Here's how the part is built. I have some questions about the finished solid (model axes, mm). A direction names the side the tool comes from. Coordinates: 2 decimals unless noted, no trailing zeros. Write each loop counter-clockwise with the first axis right and the second up, starting at its lowest first coordinate (ties: lowest second). Pieces come first, ordered by that corner, then holes.
Item 1: For faces 5 (the face through (8.25, 5.24, -0.07)), 6 (the face through (11, 16, -5)), 7 (the face through (-5, 16, 10)), which set-ups out of +Z, -Z, +X, -X, +Y, -Y let a thin tool reach every point of the face, with its end or its side?
Item 2: We'd pull the mould along X, two halves only. Please class faces 1 (the face through (-11, 16, 5)), 2 (the face through (-9.59, 22.48, -0.07)), 3 (the face through (11.49, 13.1, -0.07)), 4 (the face through (-11.46, 12.87, -0.07)): +X half, -X half, draft (parallel to the pull), parting line (faces both ways), or undercut.
Item 3: If we section it at A-A (y = -2.5): Please give me the cut outline in (x, z).
Item 4: If we section it at D-D (z = 6.25): Please give me the cut outline in (x, y).
Item 5: If we section it at B-B (x = 0): Please give me the cut outline in (y, z), then the cut area to 3 significant figures.
Item 6: If we section it at C-C (y = 13): Please give me the cut outline in (x, z).
Item 7: I'm going to push flat-ended pins straight in: pin 1 Ø2 at (y, z) = (15.5, 2) entering from +X; pin 2 Ø1.2 at (y, z) = (11, 10.5) entering from +X; pin 3 Ø0.8 at (y, z) = (18, 10) entering from -X. Where does each tip first touch, or does it pass through?
Item 8: If I drill on line 1 (Z direction, x = 0, y = 2.3); line 2 (Y direction, x = 5.5, z = 7); line 3 (X direction, y = 21, z = 4.5), over which ranges is the centre line in solid material (lowest first)?
from build123d import *

# Parameters (mm, degrees)
EXTRUDE_1582_DEPTH      = 11
EXTRUDE_1582_DEPTH_BACK = 11
EXTRUDE_2052_DEPTH      = 5
EXTRUDE_2052_DEPTH_BACK = 5
EXTRUDE_2225_DEPTH      = 5
EXTRUDE_2225_DEPTH_BACK = 5
CUT_EXTRUDE_2419_REACH  = 32.666
SKETCH_4_R              = 3.5
EXTRUDE_5_DEPTH         = 22


with BuildPart() as part:
    # Эскиз1 → Extrude 1582 (new, two sides: drawn at the far end of the back side and taken through both)
    with BuildSketch(Plane.XY.offset(-EXTRUDE_1582_DEPTH_BACK)):
        with BuildLine():
            Line((9, 0), (-9, 0))
            ThreePointArc((-9, 0), (-9.662499048, 0.250937245), (-9.992506725, 0.877809978))
            Line((-9.992506725, 0.877809978), (-10.5, 5))
            Line((-10.5, 5), (10.5, 5))
            Line((10.5, 5), (9.992506725, 0.877809978))
            ThreePointArc((9.992506725, 0.877809978), (9.662499048, 0.250937245), (9, 0))
        make_face()
    extrude(amount=EXTRUDE_1582_DEPTH + EXTRUDE_1582_DEPTH_BACK)

    # Эскиз6 → Extrude 2052 (add, two sides: drawn at the far end of the back side and taken through both)
    with BuildSketch(Plane.XY.offset(-EXTRUDE_2052_DEPTH_BACK)):
        with BuildLine():
            Line((9.000000194, 0), (-9.000000194, 0))
            ThreePointArc((-9.000000194, 0), (-9.662731652, 0.251142861), (-9.992582561, 0.87842597))
            Line((-9.992582561, 0.87842597), (-12.453151595, 20.967563779))
            ThreePointArc((-12.453151595, 20.967563779), (-12.450795845, 21.228605534), (-12.380957788, 21.480142794))
            Line((-12.380957788, 21.480142794), (-10.816937846, 25.161697034))
            ThreePointArc((-10.816937846, 25.161697034), (-10.448362214, 25.604659969), (-9.896549286, 25.770692048))
            Line((-9.896549286, 25.770692048), (-8.896549286, 25.770692048))
            Line((-8.896549286, 25.770692048), (-8.540172772, 25.153429819))
            ThreePointArc((-8.540172772, 25.153429819), (-8.5, 25), (-8.543670285, 24.847528799))
            ThreePointArc((-8.543670285, 24.847528799), (-9.603061276, 22.440310879), (-9.99820781, 19.840144231))
            ThreePointArc((-9.99820781, 19.840144231), (-10.020066103, 19.650295162), (-10.077640031, 19.468070858))
            Line((-10.077640031, 19.468070858), (-10.11018486, 19.391463424))
            ThreePointArc((-10.11018486, 19.391463424), (-10.180022917, 19.139926164), (-10.182378667, 18.878884409))
            Line((-10.182378667, 18.878884409), (-8.590049232, 5.87842597))
            ThreePointArc((-8.590049232, 5.87842597), (-8.260198323, 5.251142861), (-7.597466865, 5))
            Line((-7.597466865, 5), (7.597466865, 5))
            ThreePointArc((7.597466865, 5), (8.260198323, 5.251142861), (8.590049232, 5.87842597))
            Line((8.590049232, 5.87842597), (10.182378667, 18.878884409))
            ThreePointArc((10.182378667, 18.878884409), (10.180022917, 19.139926164), (10.11018486, 19.391463424))
            Line((10.11018486, 19.391463424), (10.077640031, 19.468070858))
            ThreePointArc((10.077640031, 19.468070858), (10.020066103, 19.650295162), (9.99820781, 19.840144231))
            ThreePointArc((9.99820781, 19.840144231), (9.603061276, 22.440310879), (8.543670285, 24.847528799))
            ThreePointArc((8.543670285, 24.847528799), (8.5, 25), (8.540172772, 25.153429819))
            Line((8.540172772, 25.153429819), (8.896549286, 25.770692048))
            Line((8.896549286, 25.770692048), (9.896549286, 25.770692048))
            ThreePointArc((9.896549286, 25.770692048), (10.448362214, 25.604659969), (10.816937846, 25.161697034))
            Line((10.816937846, 25.161697034), (12.380957788, 21.480142794))
            ThreePointArc((12.380957788, 21.480142794), (12.450795845, 21.228605534), (12.453151595, 20.967563779))
            Line((12.453151595, 20.967563779), (9.992582561, 0.87842597))
            ThreePointArc((9.992582561, 0.87842597), (9.662731652, 0.251142861), (9.000000194, 0))
        make_face()
    extrude(amount=EXTRUDE_2052_DEPTH + EXTRUDE_2052_DEPTH_BACK)

    # Эскиз3 → Extrude 2225 (add, two sides: drawn at the far end of the back side and taken through both)
    with BuildSketch(Plane(origin=(0, 0, 0), x_dir=(0, 0, -1), z_dir=(1, 0, 0)).offset(-EXTRUDE_2225_DEPTH_BACK)):
        Polygon((-9.5, 5), (-11, 5), (-11, 25.770692048), (-9.5, 24.904666645), align=None)
    extrude(amount=EXTRUDE_2225_DEPTH + EXTRUDE_2225_DEPTH_BACK)

    # Эскиз4 → Cut-Extrude 2419 (cut, up to next)
    with BuildSketch(Plane.XZ, mode=Mode.PRIVATE) as cut_extrude_2419_sk1:
        Circle(SKETCH_4_R)
    cut_extrude_2419_tool1 = extrude(cut_extrude_2419_sk1.sketch, amount=-CUT_EXTRUDE_2419_REACH, mode=Mode.PRIVATE) & part.part
    add(cut_extrude_2419_tool1.solids().sort_by_distance((0, 0, 0))[0], mode=Mode.SUBTRACT)

    # Эскиз7 → Бобышка-Вытянуть5 (add)
    with BuildSketch(Plane(origin=(0, 0, -11), x_dir=(-1, 0, 0), z_dir=(0, 0, -1))):
        with BuildLine():
            Line((7.928932188, 0), (9, 0))
            ThreePointArc((9, 0), (9.662499048, 0.250937245), (9.992506725, 0.877809978))
            Line((9.992506725, 0.877809978), (10.5, 5))
            Line((10.5, 5), (15, 5))
            ThreePointArc((15, 5), (19.330127019, -8.623724357), (7.928932188, 0))
        make_face()
        with BuildLine():
            Line((-15, 5), (-10.5, 5))
            Line((-10.5, 5), (-9.992506725, 0.877809978))
            ThreePointArc((-9.992506725, 0.877809978), (-9.662499048, 0.250937245), (-9, 0))
            Line((-9, 0), (-7.928932188, 0))
            ThreePointArc((-7.928932188, 0), (-19.330127019, -8.623724357), (-15, 5))
        make_face()
    extrude(amount=-EXTRUDE_5_DEPTH)


solid = part.part
Answer list:
1. face 5: +Z, -Z
1. face 6: -Z, +X, -X, +Y
1. face 7: +Z, -Z, -X, +Y
2. face 1: draft
2. face 2: undercut
2. face 3: +X half
2. face 4: -X half
3. outline: (-22.5, -11) - (-7.5, -11) - (-7.5, 11) - (-22.5, 11) - close; (7.5, -11) - (22.5, -11) - (22.5, 11) - (7.5, 11) - close
4. outline: (-15, 5) arc R7.5 ccw (long way) to (-7.93, 0) - (7.93, 0) arc R7.5 ccw (long way) to (15, 5) - close
5. outline: (0, -11) - (5, -11) - (5, -3.5) - (0, -3.5) - close; (0, 3.5) - (5, 3.5) - (5, 9.5) - (24.9, 9.5) - (25.77, 11) - (0, 11) - close
5. area: 106 mm2
6. outline: (-11.48, -5) - (-9.46, -5) - (-9.46, 5) - (-11.48, 5) - close; (-5, 9.5) - (5, 9.5) - (5, 11) - (-5, 11) - close; (9.46, -5) - (11.48, -5) - (11.48, 5) - (9.46, 5) - close
7. pin 1: stops at x = 11.91
7. pin 2: stops at x = 5
7. pin 3: stops at x = -5
8. line 1: z = -11 to -3.5, 3.5 to 11
8. line 2: y = 0 to 5
8. line 3: x = -12.46 to -9.91, 9.91 to 12.46
